Could you check a few things on this model? Use its own coordinates, in mm. Face numbers are marked on the shaded views. A direction names the side the tool comes from. Coordinates: 2 decimals unless noted, no trailing zeros. Order: outer loops, then holes, each group sorted by start corner. A loop starts at its lowest first (then second) coordinate and runs counter-clockwise, first axis right, second up. Notation, with made-up numbers: (-34.5, 43.25) - (4.5, 43.25) arc R7 ccw to (4.5, 56.25) - close; hole circle Ø5 at (30, -24.5). An arc over 180 degrees is marked (long way). One line per item, written item: value.
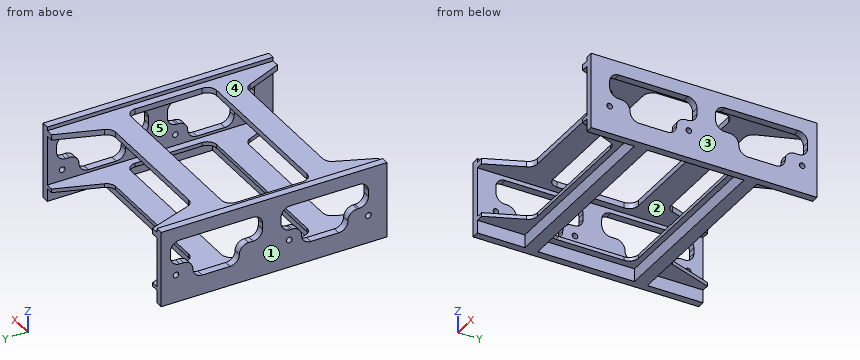
from build123d import *

# Parameters (mm, degrees)
F0_W     = 121.6
F0_H     = 41
F0_R     = 1.5
F1_DEPTH = 4
F2_W     = 121.6
F2_H     = 3
F3_DEPTH = 102
F5_DEPTH = 34.001
F6_W     = 121.6
F6_H     = 35.95
F6_R     = 1.5
F6_H_2   = 2.05
F6_H_3   = 3
F7_DEPTH = 4
F9_DEPTH = 110.001


with BuildPart() as f1:
    # F0 (on Right) → F1 (new body)
    with BuildSketch(Plane.YZ):
        with Locations((60.8, 20.5)):
            Rectangle(F0_W, F0_H)
        with Locations((10, 15)):
            Circle(F0_R, mode=Mode.SUBTRACT)
        with Locations((52.6, 15)):
            Circle(F0_R, mode=Mode.SUBTRACT)
        with Locations((113.6, 15)):
            Circle(F0_R, mode=Mode.SUBTRACT)
    extrude(amount=-F1_DEPTH)

    # F2 (on face) → F3 (join)
    with BuildSketch(Plane(origin=(-4, 0, 0), x_dir=(0, -1, 0), z_dir=(-1, 0, 0))):
        Polygon((0, 7), (0, 9), (-121.6, 9), (-121.6, 7), (-91.6, 7), (-91.6, 0), (-84.6, 0), (-84.6, 7), (-32.6, 7), (-32.6, 0), (-25.6, 0), (-25.6, 7), align=None)
        with Locations((-60.8, 37.45)):
            Rectangle(F2_W, F2_H)
    extrude(amount=F3_DEPTH)

    # F4 (on face) → F5 (cut, through all)
    with BuildSketch(Plane(origin=(0, 0, 7), x_dir=(1, 0, 0), z_dir=(0, 0, -1))):
        with BuildLine():
            Line((-8, -76.6), (-8, -40.6))
            ThreePointArc((-8, -40.6), (-9.4644660941, -37.0644660941), (-13, -35.6))
            Line((-13, -35.6), (-97, -35.6))
            ThreePointArc((-97, -35.6), (-100.5355339059, -37.0644660941), (-102, -40.6))
            Line((-102, -40.6), (-102, -76.6))
            ThreePointArc((-102, -76.6), (-100.5355339059, -80.1355339059), (-97, -81.6))
            Line((-97, -81.6), (-13, -81.6))
            ThreePointArc((-13, -81.6), (-9.4644660941, -80.1355339059), (-8, -76.6))
        make_face()
        with BuildLine():
            Line((-8, 0), (-102, 0))
            Line((-102, 0), (-93.7873133496, -19.5375492948))
            ThreePointArc((-93.7873133496, -19.5375492948), (-91.9449562371, -21.764597608), (-89.1779855536, -22.6))
            Line((-89.1779855536, -22.6), (-20.8220144464, -22.6))
            ThreePointArc((-20.8220144464, -22.6), (-18.0550437629, -21.764597608), (-16.2126866504, -19.5375492948))
            Line((-16.2126866504, -19.5375492948), (-8, 0))
        make_face()
        with BuildLine():
            Line((-8, -121.6), (-16.3246498167, -97.940468942))
            ThreePointArc((-16.3246498167, -97.940468942), (-18.1513722675, -95.5197025053), (-21.0412117709, -94.6))
            Line((-21.0412117709, -94.6), (-88.9587882291, -94.6))
            ThreePointArc((-88.9587882291, -94.6), (-91.8486277325, -95.5197025053), (-93.6753501833, -97.940468942))
            Line((-93.6753501833, -97.940468942), (-102, -121.6))
            Line((-102, -121.6), (-8, -121.6))
        make_face()
    extrude(amount=-F5_DEPTH, mode=Mode.SUBTRACT)

    # F6 (on face) → F7 (join)
    with BuildSketch(Plane(origin=(-106, 0, 0), x_dir=(0, -1, 0), z_dir=(-1, 0, 0))):
        with Locations((-60.8, 17.975)):
            Rectangle(F6_W, F6_H)
        with Locations((-113.6, 15)):
            Circle(F6_R, mode=Mode.SUBTRACT)
        with Locations((-52.6, 15)):
            Circle(F6_R, mode=Mode.SUBTRACT)
        with Locations((-10, 15)):
            Circle(F6_R, mode=Mode.SUBTRACT)
        with Locations((-60.8, 39.975)):
            Rectangle(F6_W, F6_H_2)
        with Locations((-60.8, 37.45)):
            Rectangle(F6_W, F6_H_3)
    extrude(amount=F7_DEPTH)

    # F8 (on Right) → F9 (cut, through all)
    with BuildSketch(Plane.YZ):
        with BuildLine():
            Line((52, 33.7), (15, 33.7))
            ThreePointArc((15, 33.7), (11.4644660941, 32.2355339059), (10, 28.7))
            Line((10, 28.7), (10, 25.5))
            ThreePointArc((10, 25.5), (11.4644660941, 21.9644660941), (15, 20.5))
            Line((15, 20.5), (16, 20.5))
            ThreePointArc((16, 20.5), (19.5355339059, 19.0355339059), (21, 15.5))
            ThreePointArc((21, 15.5), (22.4644660941, 11.9644660941), (26, 10.5))
            Line((26, 10.5), (41, 10.5))
            ThreePointArc((41, 10.5), (44.5355339059, 11.9644660941), (46, 15.5))
            ThreePointArc((46, 15.5), (47.4644660941, 19.0355339059), (51, 20.5))
            Line((51, 20.5), (52, 20.5))
            ThreePointArc((52, 20.5), (55.5355339059, 21.9644660941), (57, 25.5))
            Line((57, 25.5), (57, 28.7))
            ThreePointArc((57, 28.7), (55.5355339059, 32.2355339059), (52, 33.7))
        make_face()
        with BuildLine():
            Line((111.6, 33.7), (72, 33.7))
            ThreePointArc((72, 33.7), (68.4644660941, 32.2355339059), (67, 28.7))
            Line((67, 28.7), (67, 25.5))
            ThreePointArc((67, 25.5), (68.4644660941, 21.9644660941), (72, 20.5))
            Line((72, 20.5), (74.5, 20.5))
            ThreePointArc((74.5, 20.5), (78.0355339059, 19.0355339059), (79.5, 15.5))
            ThreePointArc((79.5, 15.5), (80.9644660941, 11.9644660941), (84.5, 10.5))
            Line((84.5, 10.5), (99.5, 10.5))
            ThreePointArc((99.5, 10.5), (103.0355339059, 11.9644660941), (104.5, 15.5))
            ThreePointArc((104.5, 15.5), (105.9644660941, 19.0355339059), (109.5, 20.5))
            Line((109.5, 20.5), (111.6, 20.5))
            ThreePointArc((111.6, 20.5), (115.1355339059, 21.9644660941), (116.6, 25.5))
            Line((116.6, 25.5), (116.6, 28.7))
            ThreePointArc((116.6, 28.7), (115.1355339059, 32.2355339059), (111.6, 33.7))
        make_face()
    extrude(amount=-F9_DEPTH, mode=Mode.SUBTRACT)


solid = f1.part
Item 1: Thinking about a two-plate mould opening in X: for the marked faces 1, 2 and 3, which applies, pulls with the +X half, pulls with the -X half, needs draft (parallel to the pull), parting line crosses it, or undercut?
Conclusion:
face 1: pulls with the -X half
face 2: undercut
face 3: pulls with the +X half
Item 2: I want a section at A-A on x = -75. Please give me the cut outline in (y, z).
Conclusion:
outline: (22.6, 7) - (25.6, 7) - (25.6, 0) - (32.6, 0) - (32.6, 7) - (35.6, 7) - (35.6, 9) - (22.6, 9) - close; (22.6, 35.95) - (35.6, 35.95) - (35.6, 38.95) - (22.6, 38.95) - close; (81.6, 7) - (84.6, 7) - (84.6, 0) - (91.6, 0) - (91.6, 7) - (94.6, 7) - (94.6, 9) - (81.6, 9) - close; (81.6, 35.95) - (94.6, 35.95) - (94.6, 38.95) - (81.6, 38.95) - close
Item 3: If I drill on probe 1 along Y at (x, z) = (-90.5, 4); probe 2 along Z at (x, y) = (-2.05, 113.6); probe 3 along X at (y, z) = (8, 20), over which ranges is the centre line in solid material (lowest first)?
Conclusion:
probe 1: 25.6 to 32.6, 84.6 to 91.6
probe 2: 0 to 13.5, 16.5 to 20.92, 33.28 to 41
probe 3: -110 to -106, -4 to 0
Item 4: I'm going to push flat-ended pins straight in: pin 1 Ø2 at (y, z) = (61.5, 8) entering from +X; pin 2 Ø1 at (x, z) = (-34, 4.5) entering from -Y; pin 3 Ø0.9 at (x, z) = (-69, 38) entering from -Y; pin 4 Ø2 at (x, z) = (-74.5, 8) entering from +Y. Where does each tip first touch, or does it pass through?
Conclusion:
pin 1: x = 0
pin 2: y = 25.6
pin 3: y = 22.6
pin 4: y = 94.6
Item 5: I want a section at C-C on z = 18. Please give me the cut outline in (x, y).
Conclusion:
outline: (-110, 0) - (-106, 0) - (-106, 20.33) - (-110, 20.33) - close; (-110, 46.67) - (-106, 46.67) - (-106, 78.83) - (-110, 78.83) - close; (-110, 105.17) - (-106, 105.17) - (-106, 121.6) - (-110, 121.6) - close; (-4, 0) - (0, 0) - (0, 20.33) - (-4, 20.33) - close; (-4, 46.67) - (0, 46.67) - (0, 78.83) - (-4, 78.83) - close; (-4, 105.17) - (0, 105.17) - (0, 121.6) - (-4, 121.6) - close
Item 6: I want a section at B-B on y = 106. Give the number of separate pieces and of enclosed holes in the cut face, then the cut area to 3 significant figures.
Conclusion:
separate pieces: 4
enclosed holes: 0
area: 306 mm²
Item 7: For the marked faces 4 and 5, which set-ups out of +Z, -Z, +X, -X, +Y, -Y let a thin tool reach every point of the face, with its end or its side?
Conclusion:
face 4: +Z, +Y, -Y
face 5: +Y, -Y
